```python
from build123d import *

# Parameters (mm, degrees)
CROQUIS1_W              = 16.2
CROQUIS1_H              = 9.2
CROQUIS1_W_2            = 13.2
CROQUIS1_H_2            = 6.2
SALIENTE_EXTRUIR1_DEPTH = 6.5
CROQUIS3_W              = 16.2
CROQUIS3_H              = 2.5
SALIENTE_EXTRUIR2_DEPTH = 9
CROQUIS4_R              = 1.6
CORTAR_EXTRUIR1_DEPTH   = 2.5
REDONDEO1_R             = 1
REDONDEO2_R             = 5
REDONDEO3_R             = 3
CORTAR_EXTRUIR2_REACH   = 21.538
CROQUIS5_R              = 3
CROQUIS6_R              = 2.9
CORTAR_EXTRUIR3_DEPTH   = 0.5


with BuildPart() as part:
    # Croquis1 → Saliente-Extruir1 (new body)
    with BuildSketch(Plane(origin=(0, 0, 0), x_dir=(1, 0, 0), z_dir=(0, 1, 0))):
        with Locations((6.6, 3.1)):
            Rectangle(CROQUIS1_W, CROQUIS1_H)
        with Locations((6.6, 3.1)):
            Rectangle(CROQUIS1_W_2, CROQUIS1_H_2, mode=Mode.SUBTRACT)
    extrude(amount=SALIENTE_EXTRUIR1_DEPTH)

    # Croquis3 → Saliente-Extruir2 (add)
    with BuildSketch(Plane.XZ):
        with Locations((6.6, 0.25)):
            Rectangle(CROQUIS3_W, CROQUIS3_H)
    extrude(amount=SALIENTE_EXTRUIR2_DEPTH)

    # Croquis4 → Cortar-Extruir1 (cut)
    with BuildSketch(Plane(origin=(0, 0, -1), x_dir=(-1, 0, 0), z_dir=(0, 0, -1))):
        with Locations((-6.6, -5)):
            Circle(CROQUIS4_R)
    extrude(amount=-CORTAR_EXTRUIR1_DEPTH, mode=Mode.SUBTRACT)

    # Redondeo1
    redondeo1_edges = [part.edges().sort_by_distance(p)[0] for p in [
        (-1.5, 3.25, -7.7),
        (14.7, 3.25, -7.7),
    ]]
    fillet(redondeo1_edges, radius=REDONDEO1_R)

    # Redondeo2
    redondeo2_edges = [part.edges().sort_by_distance(p)[0] for p in [
        (14.7, -9, 0.25),
        (-1.5, -9, 0.25),
    ]]
    fillet(redondeo2_edges, radius=REDONDEO2_R)

    # Redondeo3
    redondeo3_edges = [part.edges().sort_by_distance(p)[0] for p in [
        (13.95, 0, -1),
        (-0.75, 0, -1),
    ]]
    fillet(redondeo3_edges, radius=REDONDEO3_R)

    # Cortar-Extruir2: up to this face of the body (flat: up to its plane)
    cortar_extruir2_end = Plane(part.part.faces().sort_by_distance((6.6, -0.813832354, 1.5))[0])
    # Croquis5 → Cortar-Extruir2 (cut, up to the picked face)
    with BuildSketch(Plane(origin=(0, 0, -7.7), x_dir=(-1, 0, 0), z_dir=(0, 0, -1)), mode=Mode.PRIVATE) as cortar_extruir2_sk1:
        with Locations((-16.35, -3.35)):
            Circle(CROQUIS5_R)
    cortar_extruir2_tool1 = split(extrude(cortar_extruir2_sk1.sketch, amount=-CORTAR_EXTRUIR2_REACH, mode=Mode.PRIVATE), bisect_by=cortar_extruir2_end, keep=Keep.BOTH, mode=Mode.PRIVATE)
    # Croquis5 → Cortar-Extruir2 (cut, up to the picked face)
    with BuildSketch(Plane(origin=(0, 0, -7.7), x_dir=(-1, 0, 0), z_dir=(0, 0, -1)), mode=Mode.PRIVATE) as cortar_extruir2_sk2:
        with Locations((3.65, -3.35)):
            Circle(CROQUIS5_R)
    cortar_extruir2_tool2 = split(extrude(cortar_extruir2_sk2.sketch, amount=-CORTAR_EXTRUIR2_REACH, mode=Mode.PRIVATE), bisect_by=cortar_extruir2_end, keep=Keep.BOTH, mode=Mode.PRIVATE)
    add(cortar_extruir2_tool1.solids().sort_by(Axis((16.35, -3.35, -7.7), (0, 0, 1)))[0], mode=Mode.SUBTRACT)
    add(cortar_extruir2_tool2.solids().sort_by(Axis((-3.65, -3.35, -7.7), (0, 0, 1)))[0], mode=Mode.SUBTRACT)

    # Croquis6 → Cortar-Extruir3 (cut)
    with BuildSketch(Plane(origin=(0, 0, -1), x_dir=(-1, 0, 0), z_dir=(0, 0, -1))):
        with Locations((-6.6, -5)):
            Circle(CROQUIS6_R)
    extrude(amount=-CORTAR_EXTRUIR3_DEPTH, mode=Mode.SUBTRACT)


solid = part.part
```
Geometry: final body of the model. Coordinates: model frame, mm. A direction names the side the tool comes from. Give positions to 0.01 mm unless a question says otherwise; leave off trailing zeros. Write each loop counter-clockwise with the first axis right and the second up, starting at its lowest first coordinate (ties: lowest second). Pieces come first, ordered by that corner, then holes.
1. Section query B-B, the plane y = 0.5. Return loops of the section in (x, z).
2. Draft query along Z for faces 1 (the flat face through (6.5, 0, -0.5)), 2 (the cylindrical face through (-0.74, -0.562, -2.252)), 3 (the flat face through (6, 0, -7)), 4 (the flat face through (13.2, 3, -3)). Return one class per face: released by +Z, released by -Z, zero draft, split by the parting line, or undercut.
3. Section query C-C, the plane z = 0.25. Return loops of the section in (x, y), then the cut area to 3 significant figures.
4. Pin query (flat end, axial travel): P1, Ø3, axis at x = 3.5, z = -5, coming from the -Y side; P2, Ø1.7, axis at x = 6.5, y = -6, coming from the -Z side; P3, Ø0.5, axis at x = 8, z = -0.5, coming from the +Y side. Return the tip coordinate at first contact, or that it passes through.
5. Reachability of faces 5 (the flat face through (0, 3, -3)), 6 (the flat face through (5, -6, -0.5)), 7 (the flat face through (7, 3, -7.7)) from +Z, -Z, +X, -X, +Y, -Y: full face, straight path, thin tool, end or side. Return the list, or none.
6. Section query A-A, the plane x = 6.6. Return loops of the section in (y, z).
7. Line query: probe 1 along Z at (x, y) = (10.75, 1.75); probe 2 along Y at (x, z) = (6.6, 0.75); probe 3 along X at (y, z) = (0.25, -4). Output: solid intervals per line, ascending.
8. Section query D-D, the plane y = -5. Return loops of the section in (x, z), then the cut area to 3 significant figures.
Computed:
1. outline: (-1.5, -6.7) arc R1 ccw to (-0.5, -7.7) - (13.7, -7.7) arc R1 ccw to (14.7, -6.7) - (14.7, 1.5) - (-1.5, 1.5) - close; hole (0, -6.2) - (13.2, -6.2) - (13.2, 0) - (0, 0) - close
2. face 1: undercut
2. face 2: released by -Z
2. face 3: zero draft
2. face 4: undercut
3. outline: (-1.5, -1.26) arc R3 cw to (-1.34, -5.26) arc R5 ccw to (3.5, -9) - (9.7, -9) arc R5 ccw to (14.42, -5.65) arc R3 cw to (14.7, -0.84) - (14.7, 6.5) - (-1.5, 6.5) - close; hole circle Ø3.2 at (6.6, -5)
3. area: 225 mm2
4. P1: stops at y = 0
4. P2: stops at z = -0.5
4. P3: stops at y = 0
5. face 5: +Y
5. face 6: -Z
5. face 7: -Z, +X, -X, +Y, -Y
6. outline: (-9, -1) - (-7.9, -1) - (-7.9, -0.5) - (-6.6, -0.5) - (-6.6, 1.5) - (-9, 1.5) - close; (-3.4, -0.5) - (-2.1, -0.5) - (-2.1, -1) - (0, -1) - (0, 0) - (6.5, 0) - (6.5, 1.5) - (-3.4, 1.5) - close; (0, -7.7) - (6.5, -7.7) - (6.5, -6.2) - (0, -6.2) - close
7. probe 1: z = -7.7 to -6.2, 0 to 1.5
7. probe 2: y = -9 to -6.6, -3.4 to 6.5
7. probe 3: x = -1.5 to 0, 13.2 to 14.7
8. outline: (-1.14, -1) - (3.7, -1) - (3.7, -0.5) - (5, -0.5) - (5, 1.5) - (-1.14, 1.5) - close; (8.2, -0.5) - (9.5, -0.5) - (9.5, -1) - (13.84, -1) - (13.84, 1.5) - (8.2, 1.5) - close
8. area: 28.2 mm2
